Geometry check sheet. Reference: the model listing, model coordinates, mm. Face numbers are marked on the shaded views. A direction names the side the tool comes from. Give positions to 0.01 mm unless a question says otherwise; leave off trailing zeros. Order: outer loops, then holes, each group sorted by start corner. A loop starts at its lowest first (then second) coordinate and runs counter-clockwise, first axis right, second up.
from build123d import *

# Parameters (mm, degrees)
RESSALTO_EXTRUS_O1_DEPTH = 12.3
ESBO_O2_R                = 1.75
CORTE_EXTRUS_O1_DEPTH    = 22.3
CORTE_EXTRUS_O2_DEPTH    = 32.3


with BuildPart() as part:
    # Esboço1 → Ressalto-extrusão1 (new body)
    with BuildSketch(Plane.XY):
        Polygon((-14.1, 13), (-14.1, 11.4), (-14.5, 11.4), (-14.5, 1.5), (-22, 1.5), (-22, 0), (-14.5, 0), (14.5, 0), (22, 0), (22, 1.5), (14.5, 1.5), (14.5, 11.4), (14.1, 11.4), (14.1, 13), (-2.6, 13), (-2.6, 11.4), (-6.6, 11.4), (-6.6, 13), align=None)
    extrude(amount=RESSALTO_EXTRUS_O1_DEPTH)

    # Esboço2 → Corte-extrusão1 (cut)
    with BuildSketch(Plane(origin=(0, 13, 0), x_dir=(1, 0, 0), z_dir=(0, 1, 0))):
        with BuildLine():
            ThreePointArc((-18.3, -9.85), (-20.91629509, -8.76629509), (-22, -6.15))
            Line((-22, -6.15), (-22, -12.3))
            Line((-22, -12.3), (-14.5, -12.3))
            Line((-14.5, -12.3), (-14.5, -9.85))
            Line((-14.5, -9.85), (-18.3, -9.85))
        make_face()
        with BuildLine():
            ThreePointArc((-22, -6.15), (-20.91629509, -3.53370491), (-18.3, -2.45))
            Line((-18.3, -2.45), (-14.5, -2.45))
            Line((-14.5, -2.45), (-14.5, 0))
            Line((-14.5, 0), (-22, 0))
            Line((-22, 0), (-22, -6.15))
        make_face()
        with BuildLine():
            ThreePointArc((18.3, -2.45), (20.91629509, -3.53370491), (22, -6.15))
            Line((22, -6.15), (22, 0))
            Line((22, 0), (14.5, 0))
            Line((14.5, 0), (14.5, -2.45))
            Line((14.5, -2.45), (18.3, -2.45))
        make_face()
        with BuildLine():
            Line((14.5, -12.3), (22, -12.3))
            Line((22, -12.3), (22, -6.15))
            ThreePointArc((22, -6.15), (20.91629509, -8.76629509), (18.3, -9.85))
            Line((18.3, -9.85), (14.5, -9.85))
            Line((14.5, -9.85), (14.5, -12.3))
        make_face()
        with Locations((-18.3, -6.15)):
            Circle(ESBO_O2_R)
        with Locations((18.3, -6.15)):
            Circle(ESBO_O2_R)
    extrude(amount=-CORTE_EXTRUS_O1_DEPTH, mode=Mode.SUBTRACT)

    # Esboço3 → Corte-extrusão2 (cut)
    with BuildSketch(Plane.ZY.offset(14.5)):
        Polygon((2.7, 13), (2.7, 11.4), (2, 11.4), (2, 7.1), (0, 7.1), (0, 13), align=None)
        Polygon((12.3, 13), (12.3, 7.1), (10.3, 7.1), (10.3, 11.4), (9.6, 11.4), (9.6, 13), align=None)
    extrude(amount=-CORTE_EXTRUS_O2_DEPTH, mode=Mode.SUBTRACT)


solid = part.part
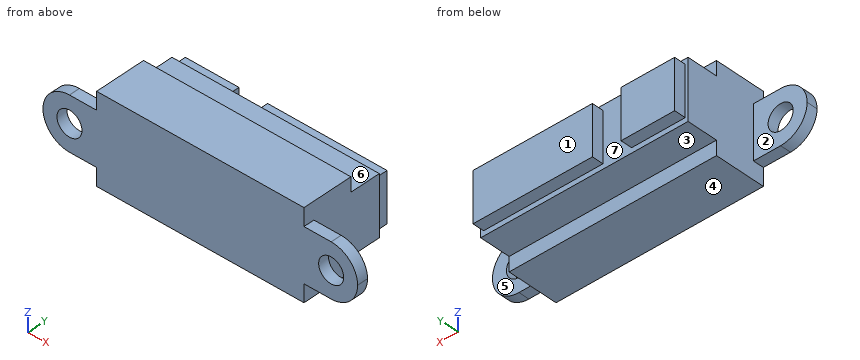
Item 1: Draft check along X on the marked faces 6 and 7. Enter one of: released by +X, released by -X, zero draft, split by the parting line, or undercut.
Reported:
face 6: zero draft
face 7: undercut
Item 2: Scan lines: L1, parallel to X at y = 0.35, z = 6.15; L2, parallel to Z at x = -18.3, y = 0.55; L3, parallel to X at y = 3, z = 1.5. Record each from-to range of solid material in increasing order.
Reported:
L1: x = -22 to -20.05, -16.55 to 16.55, 20.05 to 22
L2: z = 2.45 to 4.4, 7.9 to 9.85
L3: x = -14.5 to 14.5
Item 3: Gauge pin test, flat ends, axial feed: pin 1 (4 mm diameter, centred on x = -12.5, z = 10.5, fed in from +Y); pin 2 (4 mm diameter, centred on x = 18.3, z = 6.15, fed in from +Y); pin 3 (1.8 mm diameter, centred on x = 6.5, y = 12.5, fed in from -Z); pin 4 (3 mm diameter, centred on y = 11, z = 5, fed in from -X). Record the tip position at first contact, or that the pin passes through.
Reported:
pin 1: stops at y = 13
pin 2: stops at y = 1.5
pin 3: stops at z = 2.7
pin 4: stops at x = -14.5
Item 4: Sectioned sample at D-D (y = 7.5). Enter the section's corners in (x, z).
Reported:
outline: (-14.5, 2) - (14.5, 2) - (14.5, 10.3) - (-14.5, 10.3) - close
Item 5: Sectioned sample at B-B (x = 13). Enter the section's corners in (y, z), and give its area (3 significant figures).
Reported:
outline: (0, 0) - (7.1, 0) - (7.1, 2) - (11.4, 2) - (11.4, 2.7) - (13, 2.7) - (13, 9.6) - (11.4, 9.6) - (11.4, 10.3) - (7.1, 10.3) - (7.1, 12.3) - (0, 12.3) - close
area: 134 mm2
Item 6: Sectioned sample at A-A (z = 7). Enter the section's corners in (x, y), and give its area (3 significant figures).
Reported:
outline: (-21.9, 0) - (-19.83, 0) - (-19.83, 1.5) - (-21.9, 1.5) - close; (-16.77, 0) - (16.77, 0) - (16.77, 1.5) - (14.5, 1.5) - (14.5, 11.4) - (14.1, 11.4) - (14.1, 13) - (-2.6, 13) - (-2.6, 11.4) - (-6.6, 11.4) - (-6.6, 13) - (-14.1, 13) - (-14.1, 11.4) - (-14.5, 11.4) - (-14.5, 1.5) - (-16.77, 1.5) - close; (19.83, 0) - (21.9, 0) - (21.9, 1.5) - (19.83, 1.5) - close
area: 382 mm2
Item 7: Set-up check for the marked faces 1, 2, 3, 4 and 5: record each of +Z, -Z, +X, -X, +Y, -Y from which the full face is reachable in a straight line by a thin tool's end or side.
Reported:
face 1: +Z, -Z, +X, -X, +Y
face 2: +Z, -Z, -X, +Y
face 3: -Z, +X, -X, +Y
face 4: -Z, +X, -X, +Y, -Y
face 5: +Z, -Z, +X, +Y
Item 8: Sectioned sample at C-C (y = 2.5). Enter the section's corners in (x, z), and give its area (3 significant figures).
Reported:
outline: (-14.5, 0) - (14.5, 0) - (14.5, 12.3) - (-14.5, 12.3) - close
area: 357 mm2
